from build123d import *

# Parameters (mm, degrees)
SKETCH1_R           = 110
SKETCH1_R_2         = 3
SKETCH1_R_3         = 7.25
BOSS_EXTRUDE1_DEPTH = 6
SKETCH3_R           = 15
BOSS_EXTRUDE2_DEPTH = 15


with BuildPart() as part:
    # Sketch1 → Boss-Extrude1 (new body)
    with BuildSketch(Plane(origin=(0, 0, 0), x_dir=(1, 0, 0), z_dir=(0, 1, 0))):
        with Locations(Location((0, 0, 0), (0, 0, 270))):
            Circle(SKETCH1_R)
        with Locations(Location((-90, 0, 0), (0, 0, 270))):
            Circle(SKETCH1_R_2, mode=Mode.SUBTRACT)
        with Locations(Location((-84.572335871, 30.781812899, 0), (0, 0, 270))):
            Circle(SKETCH1_R_2, mode=Mode.SUBTRACT)
        with Locations(Location((-68.943999881, 57.850884872, 0), (0, 0, 270))):
            Circle(SKETCH1_R_2, mode=Mode.SUBTRACT)
        with Locations(Location((-45, 77.942286341, 0), (0, 0, 270))):
            Circle(SKETCH1_R_2, mode=Mode.SUBTRACT)
        with Locations(Location((-15.62833599, 88.632697771, 0), (0, 0, 270))):
            Circle(SKETCH1_R_2, mode=Mode.SUBTRACT)
        with Locations(Location((15.62833599, 88.632697771, 0), (0, 0, 270))):
            Circle(SKETCH1_R_2, mode=Mode.SUBTRACT)
        with Locations(Location((45, 77.942286341, 0), (0, 0, 270))):
            Circle(SKETCH1_R_2, mode=Mode.SUBTRACT)
        with Locations(Location((68.943999881, 57.850884872, 0), (0, 0, 270))):
            Circle(SKETCH1_R_2, mode=Mode.SUBTRACT)
        with Locations(Location((84.572335871, 30.781812899, 0), (0, 0, 270))):
            Circle(SKETCH1_R_2, mode=Mode.SUBTRACT)
        with Locations(Location((90, 0, 0), (0, 0, 270))):
            Circle(SKETCH1_R_2, mode=Mode.SUBTRACT)
        with Locations(Location((84.572335871, -30.781812899, 0), (0, 0, 270))):
            Circle(SKETCH1_R_2, mode=Mode.SUBTRACT)
        with Locations(Location((68.943999881, -57.850884872, 0), (0, 0, 270))):
            Circle(SKETCH1_R_2, mode=Mode.SUBTRACT)
        with Locations(Location((45, -77.942286341, 0), (0, 0, 270))):
            Circle(SKETCH1_R_2, mode=Mode.SUBTRACT)
        with Locations(Location((15.62833599, -88.632697771, 0), (0, 0, 270))):
            Circle(SKETCH1_R_2, mode=Mode.SUBTRACT)
        with Locations(Location((-15.62833599, -88.632697771, 0), (0, 0, 270))):
            Circle(SKETCH1_R_2, mode=Mode.SUBTRACT)
        with Locations(Location((-45, -77.942286341, 0), (0, 0, 270))):
            Circle(SKETCH1_R_2, mode=Mode.SUBTRACT)
        with Locations(Location((-68.943999881, -57.850884872, 0), (0, 0, 270))):
            Circle(SKETCH1_R_2, mode=Mode.SUBTRACT)
        with Locations(Location((-84.572335871, -30.781812899, 0), (0, 0, 270))):
            Circle(SKETCH1_R_2, mode=Mode.SUBTRACT)
        with Locations(Location((0, 0, 0), (0, 0, 270))):
            Circle(SKETCH1_R_3, mode=Mode.SUBTRACT)
    extrude(amount=BOSS_EXTRUDE1_DEPTH)

    # Sketch3 → Boss-Extrude2 (add)
    with BuildSketch(Plane(origin=(0, 6, 0), x_dir=(1, 0, 0), z_dir=(0, 1, 0))):
        with Locations(Location((0, 0, 0), (0, 0, 270))):
            Circle(SKETCH3_R)
        Polygon((-6.062177826, 10.5), (-12.124355653, 0), (-6.062177826, -10.5), (6.062177826, -10.5), (12.124355653, 0), (6.062177826, 10.5), align=None, mode=Mode.SUBTRACT)
    extrude(amount=BOSS_EXTRUDE2_DEPTH)


solid = part.part
CAD build for the part. Positions are in the model's coordinates, mm. A direction names the side the tool comes from. Coordinates: 2 decimals unless noted, no trailing zeros. Loops run counter-clockwise (first coordinate to the right, second up) from the corner with the lowest first, then second, coordinate; pieces in that order, holes last. Notation, with made-up numbers: (-18.75, 81) - (-12.75, 81) arc R6 cw to (-12.75, 92) - close; hole circle Ø10 at (-4, 49). An arc over 180 degrees is marked (long way). Use one line per item in the form item = value. Start each with the question number.
1) Band-saw the part on D-D (z = 20). Give the cut face in (x, y).
2) Band-saw the part on B-B (z = -58). Give the cut face in (x, y), and give its area (3 significant figures).
3) Flat gauge pins, fed straight in: pin 1 (10.5 mm diameter, centred on x = 1.5, z = -3.5, fed in from +Y); pin 2 (3.5 mm diameter, centred on x = -15.63, z = -88.63, fed in from -Y); pin 3 (1.5 mm diameter, centred on x = -4, y = 4, fed in from +Z); pin 4 (9.5 mm diameter, centred on x = -1, y = 15.5, fed in from -Z). Where does each tip first touch, or does it go through?
4) Drill centre lines: L1, parallel to Z at x = 43.5, y = 1; L2, parallel to Y at x = -53.5, z = 16.5; L3, parallel to X at y = 15.5, z = -6. Where is each one in solid material? Low to high. Write a range as from..to.
5) Band-saw the part on C-C (x = 3). Give the cut face in (y, z), and give its area (3 significant figures).
6) Tool access for faces 5 (the face through (-70.09, 2.96, -55.08)), 6 (the face through (9.051, 13.395, 5.324)): list every direction of +Z, -Z, +X, -X, +Y, -Y with a clear straight run to the whole face (end or side of a thin tool).
7) Two-plate mould, pull along Z, no slides. Class faces 1 (the face through (-9.051, 13.395, -5.324)), 2 (the face through (0.66, 13.395, -14.985)), 3 (the face through (81.911, 2.958, 32.166)), 4 (the face through (-23, 6, -2)): +Z half, -Z half, draft (parallel to the pull), parting line (faces both ways), or undercut.
8) Band-saw the part on A-A (x = -45). Give the cut face in (y, z), and give its area (3 significant figures).
Check values:
q1.outline = (-108.17, 0) - (108.17, 0) - (108.17, 6) - (-108.17, 6) - close
q2.outline = (-93.47, 0) - (-71.94, 0) - (-71.94, 6) - (-93.47, 6) - close; (-65.95, 0) - (65.95, 0) - (65.95, 6) - (-65.95, 6) - close; (71.94, 0) - (93.47, 0) - (93.47, 6) - (71.94, 6) - close
q2.area = 1,050 mm2
q3.pin_1 = 6
q3.pin_2 = through
q3.pin_3 = 109.95
q3.pin_4 = -15
q4.L1 = -101.03..-80.54, -75.34..75.34, 80.54..101.03
q4.L2 = 0..6
q4.L3 = -13.75..-8.66, 8.66..13.75
q5.outline = (0, -109.96) - (6, -109.96) - (6, -14.7) - (21, -14.7) - (21, -10.5) - (6, -10.5) - (6, -6.6) - (0, -6.6) - close; (0, 6.6) - (6, 6.6) - (6, 10.5) - (21, 10.5) - (21, 14.7) - (6, 14.7) - (6, 109.96) - (0, 109.96) - close
q5.area = 1,370 mm2
q6.face_5 = +Y, -Y
q6.face_6 = +Y
q7.face_1 = undercut
q7.face_2 = parting line
q7.face_3 = undercut
q7.face_4 = draft
q8.outline = (0, -100.37) - (6, -100.37) - (6, -80.94) - (0, -80.94) - close; (0, -74.94) - (6, -74.94) - (6, 74.94) - (0, 74.94) - close; (0, 80.94) - (6, 80.94) - (6, 100.37) - (0, 100.37) - close
q8.area = 1,130 mm2
